from build123d import *

# Parameters (mm, degrees)
BOSS_EXTRUDE1_DEPTH = 6.35
SKETCH2_R           = 1.35
SKETCH2_R_2         = 1.385
CUT_EXTRUDE1_DEPTH  = 38.116505762
SKETCH3_W           = 63.5
SKETCH3_H           = 88.9
SKETCH3_W_2         = 38.321076004
SKETCH3_H_2         = 47.237540142
BOSS_EXTRUDE2_DEPTH = 6.35
SKETCH5_W           = 27.94
SKETCH5_H           = 55.88
CUT_EXTRUDE3_DEPTH  = 61.153053743
SKETCH6_R           = 3.175
CUT_EXTRUDE4_DEPTH  = 61.153053743
SKETCH7_W           = 41.724968974
SKETCH7_H           = 57.858351452
BOSS_EXTRUDE3_DEPTH = 6.35
SKETCH8_R           = 14.2875
CUT_EXTRUDE5_DEPTH  = 6.35
SKETCH10_W          = 63.5
SKETCH10_H          = 60
SKETCH10_R          = 3.175
SKETCH10_W_2        = 6.35
SKETCH10_H_2        = 6.35
BOSS_EXTRUDE4_DEPTH = 6.35
FILLET1_R           = 7.62
SKETCH11_R          = 2.794
CUT_EXTRUDE6_DEPTH  = 104.404858197


with BuildPart() as part:
    # Sketch1 → Boss-Extrude1 (new body)
    with BuildSketch(Plane.XY):
        with BuildLine():
            Line((-19.69889026, 23.2987845), (-14.850045261, 29.75147823))
            ThreePointArc((-14.850045261, 29.75147823), (-14.144755454, 30.339267512), (-13.251155001, 30.55))
            Line((-13.251155001, 30.55), (13.251155001, 30.55))
            ThreePointArc((13.251155001, 30.55), (14.144755454, 30.339267512), (14.850045261, 29.75147823))
            Line((14.850045261, 29.75147823), (19.69889026, 23.2987845))
            ThreePointArc((19.69889026, 23.2987845), (19.997074131, 22.730638521), (20.1, 22.09730627))
            Line((20.1, 22.09730627), (20.1, -22.09730627))
            ThreePointArc((20.1, -22.09730627), (19.997074131, -22.730638521), (19.69889026, -23.2987845))
            Line((19.69889026, -23.2987845), (14.850045261, -29.75147823))
            ThreePointArc((14.850045261, -29.75147823), (14.144755454, -30.339267512), (13.251155001, -30.55))
            Line((13.251155001, -30.55), (-13.251155001, -30.55))
            ThreePointArc((-13.251155001, -30.55), (-14.144755454, -30.339267512), (-14.850045261, -29.75147823))
            Line((-14.850045261, -29.75147823), (-19.69889026, -23.2987845))
            ThreePointArc((-19.69889026, -23.2987845), (-19.997074131, -22.730638521), (-20.1, -22.09730627))
            Line((-20.1, -22.09730627), (-20.1, 22.09730627))
            ThreePointArc((-20.1, 22.09730627), (-19.997074131, 22.730638521), (-19.69889026, 23.2987845))
        make_face()
    extrude(amount=-BOSS_EXTRUDE1_DEPTH)

    # Sketch2 → Cut-Extrude1 (cut, through all)
    with BuildSketch(Plane(origin=(0, 0, -6.35), x_dir=(-1, 0, 0), z_dir=(0, 0, -1))):
        with Locations((17.3, 21.9487845)):
            Circle(SKETCH2_R)
        with Locations((17.3, -0.0512155)):
            Circle(SKETCH2_R)
        with Locations((17.3, -22.0512155)):
            Circle(SKETCH2_R)
        with Locations((11, -27.75)):
            Circle(SKETCH2_R_2)
        with Locations(Location((-11, -27.75, 0), (0, 0, 180))):
            Circle(SKETCH2_R_2)
        with Locations(Location((-17.3, -22.0512155, 0), (0, 0, 180))):
            Circle(SKETCH2_R)
        with Locations(Location((-17.3, -0.0512155, 0), (0, 0, 180))):
            Circle(SKETCH2_R)
        with Locations(Location((-17.3, 21.9487845, 0), (0, 0, 180))):
            Circle(SKETCH2_R)
    extrude(amount=-CUT_EXTRUDE1_DEPTH, mode=Mode.SUBTRACT)

    # Sketch3 → Boss-Extrude2 (add)
    with BuildSketch(Plane(origin=(0, 0, -6.35), x_dir=(-1, 0, 0), z_dir=(0, 0, -1))):
        with Locations((0, -6.2452155)):
            Rectangle(SKETCH3_W, SKETCH3_H)
        Rectangle(SKETCH3_W_2, SKETCH3_H_2, mode=Mode.SUBTRACT)
    extrude(amount=-BOSS_EXTRUDE2_DEPTH)

    # Sketch5 → Cut-Extrude3 (cut, through all)
    with BuildSketch(Plane.XY):
        with Locations((0, 3.0087845)):
            Rectangle(SKETCH5_W, SKETCH5_H)
    extrude(amount=-CUT_EXTRUDE3_DEPTH, mode=Mode.SUBTRACT)

    # Sketch6 → Cut-Extrude4 (cut, through all)
    with BuildSketch(Plane(origin=(0, 0, -6.35), x_dir=(-1, 0, 0), z_dir=(0, 0, -1))):
        with Locations((25.4, 31.8547845)):
            Circle(SKETCH6_R)
        with Locations((-25.4, 31.8547845)):
            Circle(SKETCH6_R)
        with Locations((-25.4, -36.7252155)):
            Circle(SKETCH6_R)
        with Locations((25.4, -36.7252155)):
            Circle(SKETCH6_R)
    extrude(amount=-CUT_EXTRUDE4_DEPTH, mode=Mode.SUBTRACT)

    # Sketch7 → Boss-Extrude3 (add)
    with BuildSketch(Plane(origin=(0, 0, -6.35), x_dir=(-1, 0, 0), z_dir=(0, 0, -1))):
        with Locations((0, 3.16744248)):
            Rectangle(SKETCH7_W, SKETCH7_H)
    extrude(amount=-BOSS_EXTRUDE3_DEPTH)

    # Sketch8 → Cut-Extrude5 (cut)
    with BuildSketch(Plane(origin=(0, 0, -6.35), x_dir=(-1, 0, 0), z_dir=(0, 0, -1))):
        with Locations((0, 17.8847845)):
            Circle(SKETCH8_R)
    extrude(amount=-CUT_EXTRUDE5_DEPTH, mode=Mode.SUBTRACT)

    # Sketch10 → Boss-Extrude4 (add)
    with BuildSketch(Plane(origin=(0, 0, -6.35), x_dir=(-1, 0, 0), z_dir=(0, 0, -1))):
        with Locations((0, 68.2047845)):
            Rectangle(SKETCH10_W, SKETCH10_H)
        with Locations((-25.4, 86.3797845)):
            Circle(SKETCH10_R, mode=Mode.SUBTRACT)
        with Locations((-25.4, 60.9797845)):
            Circle(SKETCH10_R, mode=Mode.SUBTRACT)
        with Locations(Location((25.4, 60.9797845, 0), (0, 0, 180))):
            Circle(SKETCH10_R, mode=Mode.SUBTRACT)
        with Locations(Location((25.4, 86.3797845, 0), (0, 0, 180))):
            Circle(SKETCH10_R, mode=Mode.SUBTRACT)
        with Locations((0, 86.3797845)):
            Rectangle(SKETCH10_W_2, SKETCH10_H_2, mode=Mode.SUBTRACT)
    extrude(amount=-BOSS_EXTRUDE4_DEPTH)

    # Fillet1
    fillet1_edges = [part.edges().sort_by_distance(p)[0] for p in [
        (31.75, 98.2047845, -3.175),
        (-31.75, 98.2047845, -3.175),
        (-31.75, -50.6952155, -3.175),
        (31.75, -50.6952155, -3.175),
    ]]
    fillet(fillet1_edges, radius=FILLET1_R)

    # Sketch11 → Cut-Extrude6 (cut, through all)
    with BuildSketch(Plane.XY):
        with Locations((-22.61, 17.8847845)):
            Circle(SKETCH11_R)
        with Locations((22.61, 17.8847845)):
            Circle(SKETCH11_R)
    extrude(amount=-CUT_EXTRUDE6_DEPTH, mode=Mode.SUBTRACT)


solid = part.part
Read the model definition and answer for the solid it produces. Units are mm, in the model's axes. A direction names the side the tool comes from. Coordinates: 2 decimals unless noted, no trailing zeros. Order: outer loops, then holes, each group sorted by start corner. A loop starts at its lowest first (then second) coordinate and runs counter-clockwise, first axis right, second up. Notation, with made-up numbers: (15, 72.25) -> (35, 72.25) arc R25 cw to (35, 102.25) -> close; hole circle Ø9 at (-18, 6). An arc over 180 degrees is marked (long way). Answer as a JSON object with one key per item and string values.
1) A cutting plane is placed at B-B, the plane y = 30. Determine the outline of the cut face in (x, z).
Model answer:
{"outline": "(-31.75, -6.35) -> (-27.98, -6.35) -> (-27.98, 0) -> (-31.75, 0) -> close; (-22.82, -6.35) -> (-7.57, -6.35) -> (-7.57, 0) -> (-22.82, 0) -> close; (7.57, -6.35) -> (22.82, -6.35) -> (22.82, 0) -> (7.57, 0) -> close; (27.98, -6.35) -> (31.75, -6.35) -> (31.75, 0) -> (27.98, 0) -> close"}
2) A tool of negligible diameter and unlimited length cuts with its end or side. For faces 1 (the face through (0, 83.205, -3)), 2 (the face through (29.58, 95.91, -3.13)), from which of +Z, -Z, +X, -X, +Y, -Y can it reach the whole face along a straight path? Write none if from no direction.
Model answer:
{"face 1": "+Z, -Z", "face 2": "+Z, -Z, +X, +Y"}
3) A cutting plane is placed at A-A, the plane x = 0. Determine the outline of the cut face in (y, z).
Model answer:
{"outline": "(-50.7, -6.35) -> (3.6, -6.35) -> (3.6, 0) -> (-50.7, 0) -> close; (32.17, -6.35) -> (83.2, -6.35) -> (83.2, 0) -> (32.17, 0) -> close; (89.55, -6.35) -> (98.2, -6.35) -> (98.2, 0) -> (89.55, 0) -> close"}
4) A cutting plane is placed at D-D, the plane z = -3. State how many separate pieces and enclosed holes the cut face has, plus the area to 3 significant figures.
Model answer:
{"separate pieces": "1", "enclosed holes": "12", "area": "8,420 mm²"}
5) A cutting plane is placed at C-C, the plane x = 9. Determine the outline of the cut face in (y, z).
Model answer:
{"outline": "(-50.7, -6.35) -> (6.79, -6.35) -> (6.79, 0) -> (-50.7, 0) -> close; (28.98, -6.35) -> (98.2, -6.35) -> (98.2, 0) -> (28.98, 0) -> close"}
6) Consider line 1 along Y through (x, z) = (-22.5, -1.5); line 2 along Y through (x, z) = (-23, -5); line 3 along X through (y, z) = (33, -1). Determine where each line is inside the solid, lowest interval first. Write a range as from..to.
Model answer:
{"line 1": "y = -50.7..-38.02, -35.43..15.09, 20.68..30.56, 33.15..59.69, 62.27..85.09, 87.67..98.2", "line 2": "y = -50.7..-38.8, -34.65..15.12, 20.65..29.78, 33.93..58.9, 63.06..84.3, 88.46..98.2", "line 3": "x = -31.75..-28.36, -22.44..22.44, 28.36..31.75"}
7) The mould has two halves that part along X. Classify faces 3 (the face through (23.693, 63.657, -3.219)), 4 (the face through (3.175, 86, -3)), 5 (the face through (29.58, -48.4, -3.13)), 6 (the face through (0, 98.205, -3)): released by +X, released by -X, zero draft, split by the parting line, or undercut.
Model answer:
{"face 3": "undercut", "face 4": "undercut", "face 5": "released by +X", "face 6": "zero draft"}
